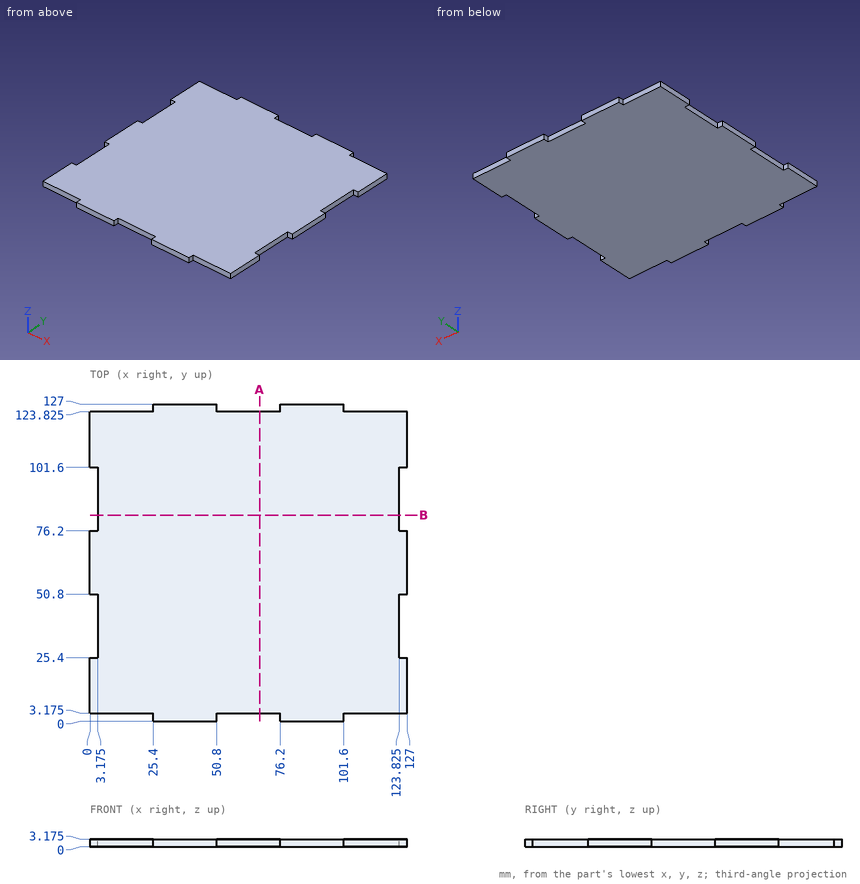
Part print with two shaded views. Sizes in mm from the minimum x, y, z corner. Round coordinates to 2 decimals unless told otherwise and drop trailing zeros. Order: outer loops, then holes, each group sorted by start corner. A loop starts at its lowest first (then second) coordinate and runs counter-clockwise, first axis right, second up. Notation, with made-up numbers: (18.5, 8) - (32.5, 8) arc R17 cw to (32.5, 28) - close; hole circle Ø6 at (1.25, 60). An arc over 180 degrees is marked (long way). Return JSON: item names as keys, results as strings.
(1) Pin check, flat tips, straight feed: pin 1 Ø1 at (x, z) = (1, 1) entering from -Y (3 decimals); pin 2 Ø1 at (x, z) = (6.5, 1.5) entering from +Y (3 decimals); pin 3 Ø1.6 at (y, z) = (124.5, 1.5) entering from +X; pin 4 Ø1.6 at (y, z) = (125, 1.5) entering from +X. Stop position of each tip, or through.
Answer key:
{"pin 1": "stops at y = 3.175", "pin 2": "stops at y = 123.825", "pin 3": "stops at x = 127", "pin 4": "stops at x = 101.6"}
(2) Cut at A-A (x = 68). Give the cut face in (y, z) (3 decimals).
Answer key:
{"outline": "(3.175, 0) - (123.825, 0) - (123.825, 3.175) - (3.175, 3.175) - close"}
(3) Wall check: probe 1 along Y at (x, z) = (116.5, 1.95) (3 decimals). Give the ranges that are in metal, low to high. Write a range as from..to.
Answer key:
{"probe 1": "y = 3.175..123.825"}
